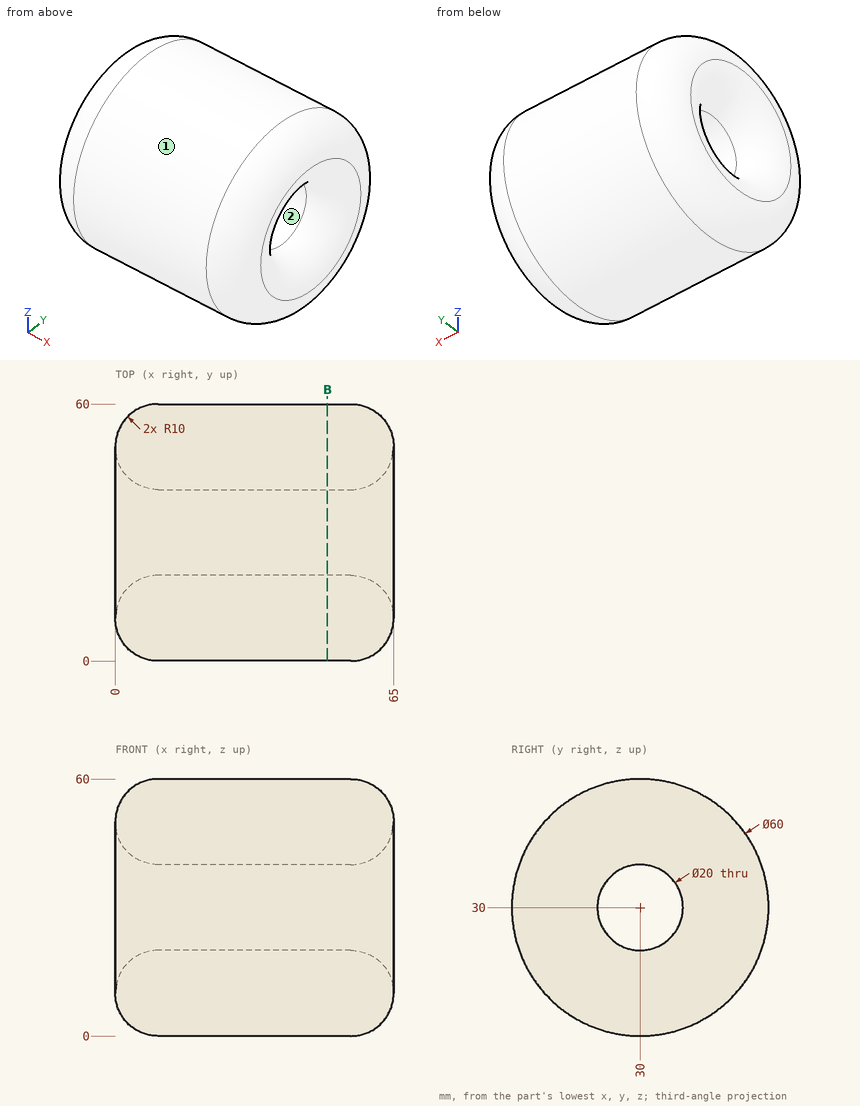
Input: dimensioned drawing with shaded views. Units: mm. Origin: part minimum x, y, z. Give positions to 0.01 mm unless a question says otherwise; leave off trailing zeros. Write each loop counter-clockwise with the first axis right and the second up, starting at its lowest first coordinate (ties: lowest second). Pieces come first, ordered by that corner, then holes.
1. First-contact query: pin 1 (3 mm diameter, centred on y = 50, z = 18, fed in from -X); pin 2 (1 mm diameter, centred on y = 9, z = 42, fed in from +X); pin 3 (2 mm diameter, centred on x = 46.5, z = 33.5, fed in from +Y); pin 4 (18 mm diameter, centred on y = 30, z = 30, fed in from -X). Flat tips, straight axial feed; report the tip coordinate or a pass-through.
2. Pull-direction query (Z, two-part tool) for the marked faces 1 and 2; classes: +Z half, -Z half, draft (parallel to the pull), parting line (faces both ways), or undercut.
3. Material intervals for line 1 along Z through (x, y) = (50, 29.5); line 2 along Z through (x, y) = (46, 22.5); line 3 along Y through (x, z) = (21, 23), sorted ascending.
4. Section query B-B (x = 49.5). Return the cut outline in (y, z), then the cut area to 3 significant figures.
Output values:
1. pin 1: stops at x = 0.17
1. pin 2: stops at x = 64.3
1. pin 3: stops at y = 59.9
1. pin 4: passes through
2. face 1: parting line
2. face 2: undercut
3. line 1: z = 0 to 20.01, 39.99 to 60
3. line 2: z = 0.95 to 23.39, 36.61 to 59.05
3. line 3: y = 0.83 to 22.86, 37.14 to 59.17
4. outline: circle Ø60 at (30, 30); hole circle Ø20 at (30, 30)
4. area: 2,510 mm2
